The listing builds one solid part. Answer for the finished solid, in the listing's coordinates (mm). A direction names the side the tool comes from. Give positions to 0.01 mm unless a question says otherwise; leave off trailing zeros. Write each loop counter-clockwise with the first axis right and the second up, starting at its lowest first coordinate (ties: lowest second). Pieces come first, ordered by that corner, then holes. Notation, with made-up numbers: (51.5, -9) - (88.5, -9) arc R29 cw to (88.5, 24) - close; hole circle Ø8 at (29.5, 17). An arc over 180 degrees is marked (long way). Write each question's results on one line, items separated by ' | '. Start each with the question number.
Q1. For a pull along Y with two mould halves and no side action, classify faces 1 (the face through (-4.19, -18.45, 0)), 2 (the face through (19.23, -0.85, -6.95)), 3 (the face through (8, -8, 104.8)), 4 (the face through (6.784, 9.115, 109.87)) as pulls with the +Y half, pulls with the -Y half, needs draft (parallel to the pull), parting line crosses it, or undercut.
Q2. Flat-ended cylindrical pins translate along their axes: pin 1 Ø5.5 at (x, y) = (-8, 8) entering from -Z; pin 2 Ø6 at (x, y) = (13.5, -11) entering from +Z; pin 3 Ø2.5 at (x, y) = (8, 8) entering from +Z; pin 4 Ø4 at (y, z) = (6, 97) entering from -X. Find the tip coordinate at first contact, or state that the pin passes through.
Q3. Section D-D (x = 12.5) is taken. Determine the outline of the cut face in (y, z), plus the area to 3 significant figures.
Q4. Find the intervals of material crossed by probe 1 along Y at (x, z) = (0, 114.45); probe 2 along Z at (x, y) = (-8.5, 17); probe 3 along Z at (x, y) = (-13, 3), in increasing order.
Q5. Section C-C (z = 12) is taken. Determine the outline of the cut face in (x, y).
Q6. Section B-B (y = 0) is taken. Determine the outline of the cut face in (x, z).
Q7. For faces 5 (the face through (0, 0, 117.3)), 6 (the face through (-9.65, -7.93, 109.87)), 7 (the face through (-12, 0, -11.7)), determine the directions among +Z, -Z, +X, -X, +Y, -Y from which every point of the face is accessible in a straight line to the end or side of a thin tool.
Q8. Section A-A (x = 0) is taken. Determine the outline of the cut face in (y, z).
Autodesk Inventor part; units mm, degrees
ref_plane "YZ Plane" through (0, 0, 0) normal (1, 0, 0) x (0, 1, 0)
ref_plane "XZ Plane" through (0, 0, 0) normal (0, 1, 0) x (-1, 0, 0)
ref_plane "XY Plane" through (0, 0, 0) normal (0, 0, 1) x (1, 0, 0)
sketch "Base" plane through (0, 0, 0) normal (0, 0, 1) x (1, 0, 0)
  circle A0 centre (0, 0) radius 18.75
  dimension "d0" = 37.5
extrude "BaseFeature" add sketch "Base" along normal blind 57
sketch "Sketch2" plane through (0, 0, 0) normal (0, 0, -1) x (-1, 0, 0)
  circle A0 centre (0, 0) radius 18.75
  circle A1 centre (0, 0) radius 19.25
  dimension "d3" = 0.5
extrude "BottomFeature" add sketch "Sketch2" along normal blind 18.2 contours A0 | A1
sketch "Panel" plane through (0, 0, -18.2) normal (0, 0, -1) x (-1, 0, 0)
  circle A0 centre (0, 0) radius 19.25
  line L0 (7.75, 17.621) -> (7.75, -17.621)
  circle A1 centre (0, 0) radius 18.75 construction
  line L1 (0, 0) -> (-19.25, 0) construction
  circle A2 centre (0, 0) radius 19.25
  line L2 (7.75, 17.621) -> (19.25, 17.621)
  line L3 (19.25, 17.621) -> (19.25, -17.621)
  line L4 (19.25, -17.621) -> (7.75, -17.621)
  line L5 (7.75, -17.621) -> (7.75, 17.621)
  dimension "d6" = 27
extrude "PanelFeature" cut sketch "Panel" against normal blind 6.5 contours A0 L0 picked at (11.5833, 0)
sketch "Gearbox" plane through (0, 0, 57) normal (0, 0, 1) x (1, 0, 0)
  circle A0 centre (0, 0) radius 16
  dimension "d9" = 32
extrude "GearboxFeature" add sketch "Gearbox" along normal blind 57.8
sketch "Shaft" plane through (0, 0, 114.8) normal (0, 0, 1) x (1, 0, 0)
  circle A0 centre (0, 0) radius 18.75
  circle A1 centre (0, 0) radius 8
  dimension "d12" = 16
extrude "ShaftFeature" cut sketch "Shaft" against normal blind 1 contours A1
sketch "MountHoles" plane through (0, 0, 114.8) normal (0, 0, 1) x (1, 0, 0)
  line L0 (0, 0) -> (-19.25, 0) construction
  line L1 (0, 0) -> (0, 19.25) construction
  circle A0 centre (0, 0) radius 19.25 construction
  line L2 (-8, -8) -> (8, -8) construction
  line L3 (8, -8) -> (8, 8) construction
  line L4 (8, 8) -> (-8, 8) construction
  line L5 (-8, 8) -> (-8, -8) construction
  circle A1 centre (-8, -8) radius 1.65
  circle A2 centre (-8, 8) radius 1.65
  circle A3 centre (8, 8) radius 1.65
  circle A4 centre (8, -8) radius 1.65
  point P0 (-8, 0)
  point P1 (0, 8)
  dimension "d16" = 16
  dimension "d17" = 3.3
extrude "MountHolesFeature" cut sketch "MountHoles" against normal blind 10
sketch "ShaftBase" plane through (0, 0, 114.8) normal (0, 0, 1) x (1, 0, 0)
  circle A0 centre (0, 0) radius 4
  dimension "d22" = 8
extrude "ShaftBaseFeature" add sketch "ShaftBase" along normal mid plane 5
properties part number "ShoulderServo"
Answers below:
1) face 1: needs draft | face 2: parting line crosses it | face 3: undercut | face 4: undercut
2) pin 1: stops at z = -18.2 | pin 2: stops at z = 114.8 | pin 3: stops at z = 104.8 | pin 4: stops at x = -15.49
3) outline: (-14.64, -18.2) - (14.64, -18.2) - (14.64, 0) - (13.98, 0) - (13.98, 57) - (9.99, 57) - (9.99, 114.8) - (-9.99, 114.8) - (-9.99, 57) - (-13.98, 57) - (-13.98, 0) - (-14.64, 0) - close | area: 3,280 mm2
4) probe 1: y = -16 to -8, -4 to 4, 8 to 16 | probe 2: z = -11.7 to 0 | probe 3: z = -11.7 to 114.8
5) outline: circle Ø37.5 at (0, 0)
6) outline: (-19.25, -11.7) - (-7.75, -11.7) - (-7.75, -18.2) - (19.25, -18.2) - (19.25, 0) - (18.75, 0) - (18.75, 57) - (16, 57) - (16, 114.8) - (8, 114.8) - (8, 113.8) - (4, 113.8) - (4, 117.3) - (-4, 117.3) - (-4, 113.8) - (-8, 113.8) - (-8, 114.8) - (-16, 114.8) - (-16, 57) - (-18.75, 57) - (-18.75, 0) - (-19.25, 0) - close
7) face 5: +Z, +X, -X, +Y, -Y | face 6: +Z | face 7: -Z, -X, +Y, -Y
8) outline: (-19.25, -18.2) - (19.25, -18.2) - (19.25, 0) - (18.75, 0) - (18.75, 57) - (16, 57) - (16, 114.8) - (8, 114.8) - (8, 113.8) - (4, 113.8) - (4, 117.3) - (-4, 117.3) - (-4, 113.8) - (-8, 113.8) - (-8, 114.8) - (-16, 114.8) - (-16, 57) - (-18.75, 57) - (-18.75, 0) - (-19.25, 0) - close
